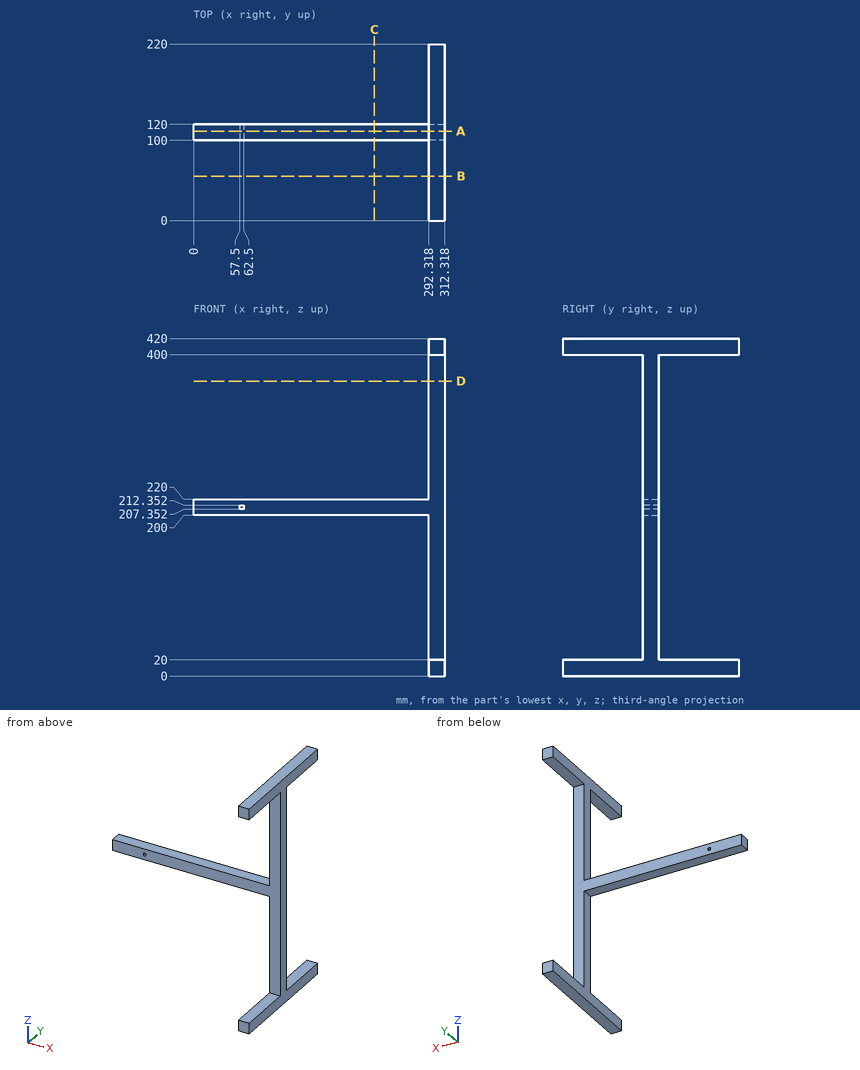
Job drawing, mm, ordinate dimensions from the low corner. One solid piece. Coordinates: 2 decimals unless noted, no trailing zeros. Order: outer loops, then holes, each group sorted by start corner. A loop starts at its lowest first (then second) coordinate and runs counter-clockwise, first axis right, second up. Notation, with made-up numbers: (87, 40) -> (110, 40) arc R21 ccw to (110, 63) -> close; hole circle Ø3 at (-19.75, 81.25). An arc over 180 degrees is marked (long way). Answer in a Markdown table with one row per item. Add a question column.
Q1. Band-saw the part on A-A, the plane y = 111.5. List the corners of the cut face in (x, z), then the cut area to 3 significant figures.
Q2. Drop flat-ended pins along their axis: pin 1 (22 mm diameter, centred on x = 90.5, y = 114, fed in from -Z); pin 2 (16 mm diameter, centred on x = 300.5, y = 170.5, fed in from -Z); pin 3 (16 mm diameter, centred on x = 217.5, y = 105, fed in from +Z). Give the stop position or say it passes through.
Q3. Wall check: line 1 along Z through (x, y) = (300, 207); line 2 along Y through (x, z) = (48.5, 200.5); line 3 along Z through (x, y) = (115.5, 119.5). Give the ranges that are in metal, low to high. Write a range as [from, to].
Q4. Band-saw the part on C-C, the plane x = 225. List the corners of the cut face in (y, z), then the cut area to 3 significant figures.
Q5. Band-saw the part on B-B, the plane y = 55.5. List the corners of the cut face in (x, z).
Q6. Band-saw the part on D-D, the plane z = 367. List the corners of the cut face in (x, y).
Answers follow:
| question | item | result |
|---|---|---|
| 1 | outline | (0, 200) -> (292.32, 200) -> (292.32, 0) -> (312.32, 0) -> (312.32, 420) -> (292.32, 420) -> (292.32, 220) -> (0, 220) -> close; hole (57.5, 207.35) -> (62.5, 207.35) -> (62.5, 212.35) -> (57.5, 212.35) -> close |
| 1 | area | 14,200 mm^2 |
| 2 | pin 1 | z = 200 |
| 2 | pin 2 | z = 0 |
| 2 | pin 3 | z = 220 |
| 3 | line 1 | [0, 20], [400, 420] |
| 3 | line 2 | [100, 120] |
| 3 | line 3 | [200, 220] |
| 4 | outline | (100, 200) -> (120, 200) -> (120, 220) -> (100, 220) -> close |
| 4 | area | 400 mm^2 |
| 5 | outline | (292.32, 0) -> (312.32, 0) -> (312.32, 20) -> (292.32, 20) -> close; (292.32, 400) -> (312.32, 400) -> (312.32, 420) -> (292.32, 420) -> close |
| 6 | outline | (292.32, 100) -> (312.32, 100) -> (312.32, 120) -> (292.32, 120) -> close |
